```python
from build123d import *

# Parameters (mm, degrees)
F1_DEPTH = 6.5
F2_R     = 1
F3_R     = 1
F4_R     = 0.99999
F5_R     = 1


# Not quite as in the source:
# - a fillet or chamfer is up to 0.001 mm smaller than in the source, because OpenCascade refuses the exact size


with BuildPart() as f1:
    # F0 (on Top) → F1 (new body)
    with BuildSketch(Plane.XY):
        Polygon((-2.3, 2.3), (2.3, 2.3), (2.3, -2.3), (1.2, -2.3), (1.2, -9.2), (3.2, -9.2), (3.2, -4.3), (4.3, -4.3), (4.3, 4.3), (-4.3, 4.3), (-4.3, 0.6), (-4.3, -0.4), (-4.3, -1.55), (-4.3, -2.3), (-4.3, -2.55), (-4.3, -9.2), (-2.3, -9.2), (-2.3, -2.3), align=None)
        with BuildLine():
            Line((-5.7826505025, -2.55), (-4.3, -2.55))
            Line((-4.3, -2.55), (-4.3, -2.3))
            Line((-4.3, -2.3), (-4.3, -1.55))
            Line((-4.3, -1.55), (-6.1404547021, -1.55))
            ThreePointArc((-6.1404547021, -1.55), (-6.8, -1.85), (-7.4595452979, -1.55))
            Line((-7.4595452979, -1.55), (-9.3, -1.55))
            Line((-9.3, -1.55), (-9.3, -2.55))
            Line((-9.3, -2.55), (-7.8173494975, -2.55))
            Line((-7.8173494975, -2.55), (-5.7826505025, -2.55))
        make_face()
        with BuildLine():
            ThreePointArc((-7.8173494975, -2.55), (-6.8, -2.85), (-5.7826505025, -2.55))
            Line((-5.7826505025, -2.55), (-7.8173494975, -2.55))
        make_face()
        with BuildLine():
            Line((-6.1404547021, -0.4), (-4.3, -0.4))
            Line((-4.3, -0.4), (-4.3, 0.6))
            Line((-4.3, 0.6), (-5.7826505025, 0.6))
            ThreePointArc((-5.7826505025, 0.6), (-6.8, 0.9), (-7.8173494975, 0.6))
            Line((-7.8173494975, 0.6), (-9.3, 0.6))
            Line((-9.3, 0.6), (-9.3, -0.4))
            Line((-9.3, -0.4), (-7.4595452979, -0.4))
            ThreePointArc((-7.4595452979, -0.4), (-6.8, -0.1), (-6.1404547021, -0.4))
        make_face()
    extrude(amount=F1_DEPTH)

    # F2
    f2_edges = [f1.edges().sort_by_distance(p)[0] for p in [
        (-7.817349, -2.55, 3.25),
        (-7.817349, 0.6, 3.25),
        (-5.782651, 0.6, 3.25),
    ]]
    fillet(f2_edges, radius=F2_R)

    # F3
    f3_edges = [f1.edges().sort_by_distance(p)[0] for p in [
        (-6.140455, -1.55, 3.25),
        (-7.459545, -1.55, 3.25),
        (-7.459545, -0.4, 3.25),
        (-6.140455, -0.4, 3.25),
    ]]
    fillet(f3_edges, radius=F3_R)

    # F4 (radius 1 in the source; OpenCascade refuses exactly that, so slightly less here)
    f4_edges = [f1.edges().sort_by_distance(p)[0] for p in [
        (-4.3, -9.2, 3.25),
        (-2.3, -9.2, 3.25),
        (1.2, -9.2, 3.25),
        (3.2, -9.2, 3.25),
        (-4.3, 4.3, 3.25),
        (4.3, -4.3, 3.25),
        (4.3, 4.3, 3.25),
        (1.2, -2.3, 3.25),
    ]]
    fillet(f4_edges, radius=F4_R)

    # F5
    f5_edges = [f1.edges().sort_by_distance(p)[0] for p in [
        (-2.3, 2.3, 3.25),
        (2.3, 2.3, 3.25),
        (2.3, -2.3, 3.25),
        (3.2, -4.3, 3.25),
        (-4.3, 0.6, 3.25),
        (-4.3, -2.55, 3.25),
        (-5.782651, -2.55, 3.25),
    ]]
    fillet(f5_edges, radius=F5_R)


solid = f1.part
```
Input: part model. Units: mm. Frame: model coordinates. A direction names the side the tool comes from. Round coordinates to 2 decimals unless told otherwise and drop trailing zeros. Loops run counter-clockwise (first coordinate to the right, second up) from the corner with the lowest first, then second, coordinate; pieces in that order, holes last. Notation, with made-up numbers: (48, 71) -> (59, 71) arc R25 cw to (59, 90) -> close; hole circle Ø9 at (80.5, 58.5). An arc over 180 degrees is marked (long way). Use one line per item in the form item = value. Start each with the question number.
Item 1: Mould query, pull axis X, two halves, no side actions, for faces 1 (the face through (-4.3, 2, 3)), 2 (the face through (-5, -0.4, 3)), 3 (the face through (1.501, -8.915, 3.296)). Classes: pulls with the +X half, pulls with the -X half, needs draft (parallel to the pull), parting line crosses it, or undercut.
Item 2: Section query D-D on y = 3.75. Return the cut outline in (x, z), then the cut area to 3 significant figures.
Item 3: Section query A-A on y = -6.75. Return the cut outline in (x, z), then the cut area to 3 significant figures.
Item 4: Section query C-C on x = 1. Return the cut outline in (y, z), then the cut area to 3 significant figures.
Item 5: Set-up query: faces 4 (the face through (-6.8, -0.1, 3.2)), 5 (the face through (-1.999, 2.015, 3.296)), 6 (the face through (-9, -2.55, 3)), 7 (the face through (-9, 0.6, 3)), 8 (the face through (-4.3, -1, 3)). Return all of +Z, -Z, +X, -X, +Y, -Y with unobstructed straight access to the full face (end or side cutting, diameter ignored); none if empty.
Item 6: Material intervals for L1, parallel to X at y = -0.5, z = 2.25; L2, parallel to X at y = -5, z = 1.75; L3, parallel to Y at x = -0.75, z = 5.5, sorted ascending. Write a range as from..to.
Item 7: Section query B-B on x = -6.75. Return the cut outline in (y, z).
Item 8: Contact query for flat-ended pins moving along their axis: pin 1 Ø1.2 at (x, z) = (-8.5, 2) entering from -Y; pin 2 Ø1.2 at (x, z) = (-8.5, 2) entering from +Y; pin 3 Ø0.7 at (x, z) = (-5.5, 2) entering from +Y. Output: stop coordinate, or through.
Ans:
q1.face_1 = pulls with the -X half
q1.face_2 = needs draft
q1.face_3 = undercut
q2.outline = (-4.19, 0) -> (4.19, 0) -> (4.19, 6.5) -> (-4.19, 6.5) -> close
q2.area = 54.5 mm^2
q3.outline = (-4.3, 0) -> (-2.3, 0) -> (-2.3, 6.5) -> (-4.3, 6.5) -> close; (1.2, 0) -> (3.2, 0) -> (3.2, 6.5) -> (1.2, 6.5) -> close
q3.area = 26.0 mm^2
q4.outline = (2.3, 0) -> (4.3, 0) -> (4.3, 6.5) -> (2.3, 6.5) -> close
q4.area = 13.0 mm^2
q5.face_4 = +Z, -Z
q5.face_5 = +Z, -Z, -Y
q5.face_6 = +Z, -Z, -X, -Y
q5.face_7 = +Z, -Z, -X, +Y
q5.face_8 = +Z, -Z, -X
q6.L1 = -4.3..-2.3, 2.3..4.3
q6.L2 = -4.3..-2.3, 1.2..3.2
q6.L3 = 2.3..4.3
q7.outline = (-2.85, 0) -> (-1.85, 0) -> (-1.85, 6.5) -> (-2.85, 6.5) -> close; (-0.1, 0) -> (0.9, 0) -> (0.9, 6.5) -> (-0.1, 6.5) -> close
q8.pin_1 = -2.57
q8.pin_2 = 0.62
q8.pin_3 = 0.66
